For this review, take the finished solid that the model builds, in its own axes (mm). Face numbers are marked on the shaded views. A direction names the side the tool comes from. Give positions to 0.01 mm unless a question says otherwise; leave off trailing zeros. Order: outer loops, then holes, each group sorted by start corner. A loop starts at its lowest first (then second) coordinate and runs counter-clockwise, first axis right, second up.
Item 1: The part is to be moulded in two halves that separate along X. For the marked faces 3, 4, 5 and 6, say which applies: released by +X, released by -X, zero draft, split by the parting line, or undercut.
Item 2: Consider section A-A (y = -29.5). Give the boundary of the cut face in (x, z).
Item 3: Consider section B-B (x = 97.5). Give the boundary of the cut face in (y, z), plus the area to 3 significant figures.
Item 4: For probe 1 along X at (y, z) = (-17, 9); probe 2 along X at (y, z) = (-37.5, 42); probe 3 along X at (y, z) = (-37, 7), list the stretches that pass through material, from the lowest coordinate up.
Item 5: For P1, Ø0.8, axis at x = 170, y = -9, coming from the +Z side; P2, Ø3, axis at x = 162, z = 24, coming from the +Y side; P3, Ø7.5, axis at x = 156, y = -19.5, coming from the -Z side; P4, Ø9, axis at x = 122.04, y = -33.04, coming from the -Z side, all flat-tipped, find the tip position at first contact; note any pin that passes through.
Item 6: Consider section C-C (z = 43.5). Give the boundary of the cut face in (x, y), plus the area to 3 significant figures.
Item 7: Machinability: for the marked faces 1 and 2, which of the approach directions +Z, -Z, +X, -X, +Y, -Y give a long, thin tool a straight path to every point of the face, cutting with its end or side? Answer none if there is none.
Item 8: Consider section D-D (z = 38). Give the boundary of the cut face in (x, y).
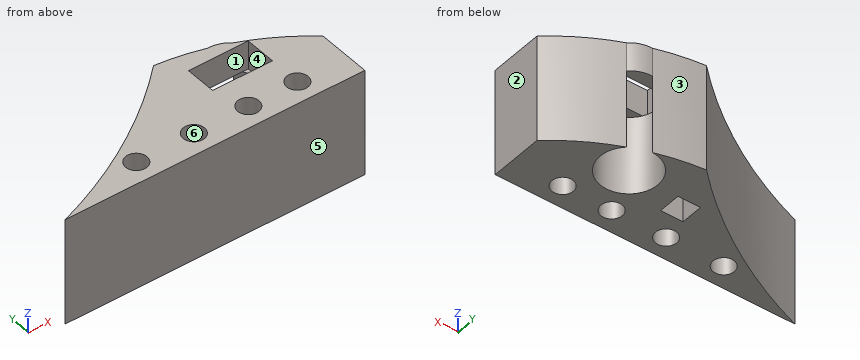
```python
from build123d import *

# Parameters (mm, degrees)
F0_R     = 5
F1_DEPTH = 50
F2_DEPTH = 36.6
F3_R     = 4.8
F4_DEPTH = 2.7
F5_W     = 10.5
F5_H     = 10.5
F6_DEPTH = 40
F7_W     = 27.904123
F7_H     = 14.441377
F8_DEPTH = 25


with BuildPart() as f1:
    # F0 (on Top) → F1 (new body)
    with BuildSketch(Plane.XY):
        with BuildLine():
            ThreePointArc((134.282529, 6.80419), (96.779809, -22.438314), (53.993077, -43.19581))
            Line((53.993077, -43.19581), (193.993077, -43.19581))
            Line((193.993077, -43.19581), (193.993077, -18.19581))
            ThreePointArc((193.993077, -18.19581), (180.440706, -8.448382), (165.548028, -0.906017))
            ThreePointArc((165.548028, -0.906017), (168.901273, -5.468336), (170.088644, -11.004504))
            ThreePointArc((170.088644, -11.004504), (147.215011, -20.719698), (156.105681, 2.486854))
            ThreePointArc((156.105681, 2.486854), (145.305567, 5.208938), (134.282529, 6.80419))
        make_face()
        with Locations((95.127106, -33.044094)):
            Circle(F0_R, mode=Mode.SUBTRACT)
        with Locations((122.039258, -33.044094)):
            Circle(F0_R, mode=Mode.SUBTRACT)
        with Locations((147.4967, -33.044094)):
            Circle(F0_R, mode=Mode.SUBTRACT)
        with Locations((170.408398, -33.044094)):
            Circle(F0_R, mode=Mode.SUBTRACT)
        with BuildLine():
            ThreePointArc((165.548028, -0.906017), (161.153764, 1.700207), (156.105681, 2.486854))
            ThreePointArc((156.105681, 2.486854), (147.215011, -20.719698), (170.088644, -11.004504))
            ThreePointArc((170.088644, -11.004504), (168.901273, -5.468336), (165.548028, -0.906017))
        make_face()
    extrude(amount=F1_DEPTH)

    # F0 (on Top) → F2 (cut)
    with BuildSketch(Plane.XY):
        with BuildLine():
            ThreePointArc((165.548028, -0.906017), (161.153764, 1.700207), (156.105681, 2.486854))
            ThreePointArc((156.105681, 2.486854), (147.215011, -20.719698), (170.088644, -11.004504))
            ThreePointArc((170.088644, -11.004504), (168.901273, -5.468336), (165.548028, -0.906017))
        make_face()
    extrude(amount=F2_DEPTH, mode=Mode.SUBTRACT)

    # F3 (on face) → F4 (cut)
    with BuildSketch(Plane(origin=(0, 0, 36.6), x_dir=(1, 0, 0), z_dir=(0, 0, -1))):
        with Locations((156.588644, 11.004504)):
            Circle(F3_R)
    extrude(amount=-F4_DEPTH, mode=Mode.SUBTRACT)

    # F5 (on face) → F6 (cut)
    with BuildSketch(Plane.XY):
        with Locations((127.963409, -16.812982)):
            Rectangle(F5_W, F5_H)
    extrude(amount=F6_DEPTH, mode=Mode.SUBTRACT)

    # F7 (on face) → F8 (cut)
    with BuildSketch(Plane(origin=(0, 0, 36.6), x_dir=(1, 0, 0), z_dir=(0, 0, -1))):
        with Locations((156.589418, 10.691026)):
            Rectangle(F7_W, F7_H)
    extrude(amount=-F8_DEPTH, mode=Mode.SUBTRACT)


solid = f1.part
```
Resolved:
1. face 3: released by +X
1. face 4: undercut
1. face 5: zero draft
1. face 6: undercut
2. outline: (84.61, 0) - (91.6, 0) - (91.6, 50) - (84.61, 50) - close; (98.65, 0) - (118.51, 0) - (118.51, 50) - (98.65, 50) - close; (125.57, 0) - (143.97, 0) - (143.97, 50) - (125.57, 50) - close; (151.02, 0) - (166.88, 0) - (166.88, 50) - (151.02, 50) - close; (173.94, 0) - (193.99, 0) - (193.99, 50) - (173.94, 50) - close
3. outline: (-43.2, 0) - (-37.45, 0) - (-37.45, 50) - (-43.2, 50) - close; (-28.64, 0) - (-21.99, 0) - (-21.99, 50) - (-28.64, 50) - close
3. area: 620 mm2
4. probe 1: x = 105.1 to 122.71, 133.21 to 144.49, 168.68 to 192.55
4. probe 2: x = 68.24 to 92.86, 97.4 to 119.77, 124.31 to 145.23, 149.76 to 168.14, 172.68 to 193.99
4. probe 3: x = 69.37 to 92.07, 98.19 to 118.98, 125.1 to 144.44, 150.55 to 167.35, 173.47 to 193.99
5. P1: stops at z = 36.6
5. P2: stops at y = -22.6
5. P3: stops at z = 36.6
5. P4: passes through
6. outline: (53.99, -43.2) - (193.99, -43.2) - (193.99, -18.2) arc R108 ccw to (165.55, -0.91) arc R13.5 ccw to (156.11, 2.49) arc R108 ccw to (134.28, 6.8) arc R226.25 cw to start; hole circle Ø10 at (95.13, -33.04); hole circle Ø10 at (122.04, -33.04); hole circle Ø10 at (147.5, -33.04); hole (142.64, -17.91) - (170.54, -17.91) - (170.54, -3.47) - (142.64, -3.47) - close; hole circle Ø10 at (170.41, -33.04)
6. area: 3,430 mm2
7. face 1: +Z
7. face 2: +Z, -Z, +X, +Y, -Y
8. outline: (53.99, -43.2) - (193.99, -43.2) - (193.99, -18.2) arc R108 ccw to (165.55, -0.91) arc R13.5 ccw to (156.11, 2.49) arc R108 ccw to (134.28, 6.8) arc R226.25 cw to start; hole circle Ø10 at (95.13, -33.04); hole circle Ø10 at (122.04, -33.04); hole (122.71, -22.06) - (133.21, -22.06) - (133.21, -11.56) - (122.71, -11.56) - close; hole circle Ø10 at (147.5, -33.04); hole (142.64, -17.91) - (170.54, -17.91) - (170.54, -3.47) - (142.64, -3.47) - close; hole circle Ø10 at (170.41, -33.04)
